Geometry: final body of the model. Coordinates: model frame, mm. Face numbers are marked on the shaded views. Give positions to 0.01 mm unless a question says otherwise; leave off trailing zeros. Loops run counter-clockwise (first coordinate to the right, second up) from the corner with the lowest first, then second, coordinate; pieces in that order, holes last. Notation, with made-up numbers: (57.5, 51) -> (77.5, 51) arc R25 ccw to (77.5, 84) -> close; hole circle Ø11 at (9.5, -2.5). An arc over 180 degrees is marked (long way). One line per question, with ' | ' between items. Start each with the question number.
Item 1: Material intervals for line 1 along Z through (x, y) = (9.25, 0.25); line 2 along Z through (x, y) = (16.5, 2.3); line 3 along Z through (x, y) = (15.5, 1.65), sorted ascending. Write a range as [from, to].
Item 2: Section A-A on y = 1.55. Give the number of separate pieces and of enclosed holes in the cut face, then the cut area to 3 significant figures.
Item 3: Section B-B on x = 15. Return loops of the section in (y, z), then the cut area to 3 significant figures.
Item 4: Mould query, pull axis Y, two halves, no side actions, for the marked faces 1 and 2. Classes: released by +Y, released by -Y, zero draft, split by the parting line, or undercut.
Item 5: Pin query (flat end, axial travel): P1, Ø2.5, axis at x = 15.08, z = 18.83, coming from the -Y side. Return the tip coordinate at first contact, or that it passes through.
from build123d import *

# Parameters (mm, degrees)
SKETCH1_W           = 19.05
SKETCH1_H           = 2.38125
BOSS_EXTRUDE1_DEPTH = 88.9
SKETCH5_R           = 1.905
CUT_EXTRUDE4_DEPTH  = 3.38125
SKETCH9_W           = 19.05
SKETCH9_H           = 29.6545
BOSS_EXTRUDE4_DEPTH = 2.38125
BOSS_EXTRUDE5_DEPTH = 2.38125
SKETCH11_R          = 1.905
CUT_EXTRUDE6_DEPTH  = 2.54
SKETCH12_W          = 19.05
SKETCH12_H          = 29.6545
CUT_EXTRUDE7_DEPTH  = 3.38125


with BuildPart() as part:
    # Sketch1 → Boss-Extrude1 (new body)
    with BuildSketch(Plane.XY):
        with Locations((9.525, 1.190625)):
            Rectangle(SKETCH1_W, SKETCH1_H)
    extrude(amount=BOSS_EXTRUDE1_DEPTH)

    # Sketch5 → Cut-Extrude4 (cut, through all)
    with BuildSketch(Plane(origin=(0, 2.38125, 0), x_dir=(1, 0, 0), z_dir=(0, 1, 0))):
        with Locations((15.08125, -39.14775)):
            Circle(SKETCH5_R)
        with Locations((15.08125, -18.82775)):
            Circle(SKETCH5_R)
        Polygon((16.317595, -28.98775), (16.317595, -32.5755), (15.08125, -32.5755), (13.844905, -32.5755), (13.844905, -25.2095), (16.317595, -25.2095), align=None)
        Polygon((15.08125, -52.8955), (16.317595, -52.8955), (16.317595, -45.5295), (13.844905, -45.5295), (13.844905, -52.8955), align=None)
    extrude(amount=-CUT_EXTRUDE4_DEPTH, mode=Mode.SUBTRACT)

    # Sketch9 → Boss-Extrude4 (add)
    with BuildSketch(Plane(origin=(0, 2.38125, 0), x_dir=(1, 0, 0), z_dir=(0, 1, 0))):
        with Locations((9.525, 14.82725)):
            Rectangle(SKETCH9_W, SKETCH9_H)
    extrude(amount=-BOSS_EXTRUDE4_DEPTH)

    # Sketch8 → Boss-Extrude5 (add)
    with BuildSketch(Plane(origin=(0, 2.38125, 0), x_dir=(1, 0, 0), z_dir=(0, 1, 0))):
        Polygon((19.05, -88.9), (0, -88.9), (0, -114.3), (0, -120.65), (19.05, -120.65), (19.05, -114.3), align=None)
    extrude(amount=-BOSS_EXTRUDE5_DEPTH)

    # Sketch11 → Cut-Extrude6 (cut)
    with BuildSketch(Plane(origin=(0, 2.38125, 0), x_dir=(1, 0, 0), z_dir=(0, 1, 0))):
        with Locations((9.525, -113.919)):
            Circle(SKETCH11_R)
        with Locations((9.525, -93.3958)):
            Circle(SKETCH11_R)
    extrude(amount=-CUT_EXTRUDE6_DEPTH, mode=Mode.SUBTRACT)

    # Sketch12 → Cut-Extrude7 (cut, through all)
    with BuildSketch(Plane(origin=(0, 2.38125, 0), x_dir=(1, 0, 0), z_dir=(0, 1, 0))):
        with Locations((9.525, 14.82725)):
            Rectangle(SKETCH12_W, SKETCH12_H)
    extrude(amount=-CUT_EXTRUDE7_DEPTH, mode=Mode.SUBTRACT)


solid = part.part
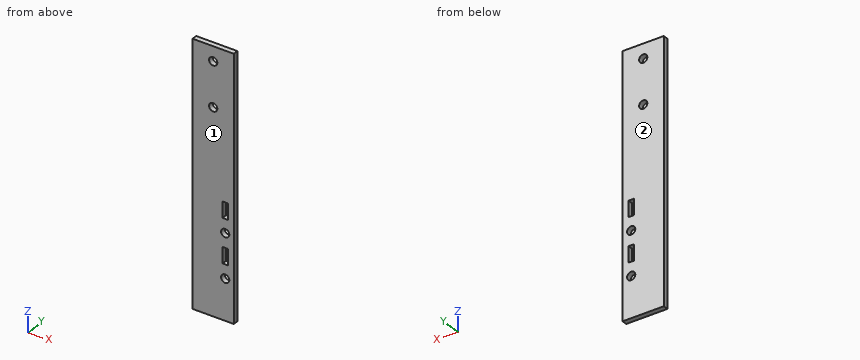
Result sheet:
1) line 1: z = [0, 91.51], [95.28, 112.03], [115.8, 120.65] | line 2: z = [0, 17.56], [20.1, 37.88], [40.42, 120.65] | line 3: z = [0, 16.97], [20.69, 25.21], [32.58, 37.29], [41.01, 45.53], [52.9, 120.65]
2) separate pieces: 1 | enclosed holes: 6 | area: 2,220 mm²
3) outline: (0, 0) -> (2.38, 0) -> (2.38, 16.92) -> (0, 16.92) -> close; (0, 20.73) -> (2.38, 20.73) -> (2.38, 25.21) -> (0, 25.21) -> close; (0, 32.58) -> (2.38, 32.58) -> (2.38, 37.24) -> (0, 37.24) -> close; (0, 41.05) -> (2.38, 41.05) -> (2.38, 45.53) -> (0, 45.53) -> close; (0, 52.9) -> (2.38, 52.9) -> (2.38, 120.65) -> (0, 120.65) -> close | area: 234 mm²
4) face 1: released by -Y | face 2: released by +Y
5) P1: passes through
